Answer from the drawing. Dimensions are ordinates in mm from the lowest x, y and z of the part. Coordinates: 2 decimals unless noted, no trailing zeros. Write each loop counter-clockwise with the first axis right and the second up, starting at its lowest first coordinate (ties: lowest second). Pieces come first, ordered by that corner, then holes.
(1) The part is cut by section B-B, the plane z = 1.5. Determine the outline of the cut face in (x, y).
(2) The part is cut by section C-C, the plane y = 2.15. Determine the outline of the cut face in (x, z).
(3) Given pin 1 (8 mm diameter, centred on x = 18, z = 11.5, fed in from -Y); pin 2 (1.5 mm diameter, centred on x = 49, y = 1, fed in from -Z); pin 3 (0.9 mm diameter, centred on y = 1, z = 1, fed in from +X); pin 4 (1.5 mm diameter, centred on x = 16.5, y = 1.5, fed in from -Z), each flat-ended and moving along its own axis, determine where each tip first touches the part or whether it passes through.
(4) The part is cut by section D-D, the plane x = 25.4. Determine the outline of the cut face in (y, z), and give its area (3 significant figures).
(5) Straight lines are drawn through the part: line 1 along X through (y, z) = (1, 1.5); line 2 along Z through (x, y) = (49.3, 1.05); line 3 along X through (y, z) = (0.25, 4.25). For each, find the intervals that lie inside material, in ascending order.
(6) The part is cut by section A-A, the plane x = 49.3. Determine the outline of the cut face in (y, z), and give its area (3 significant figures).
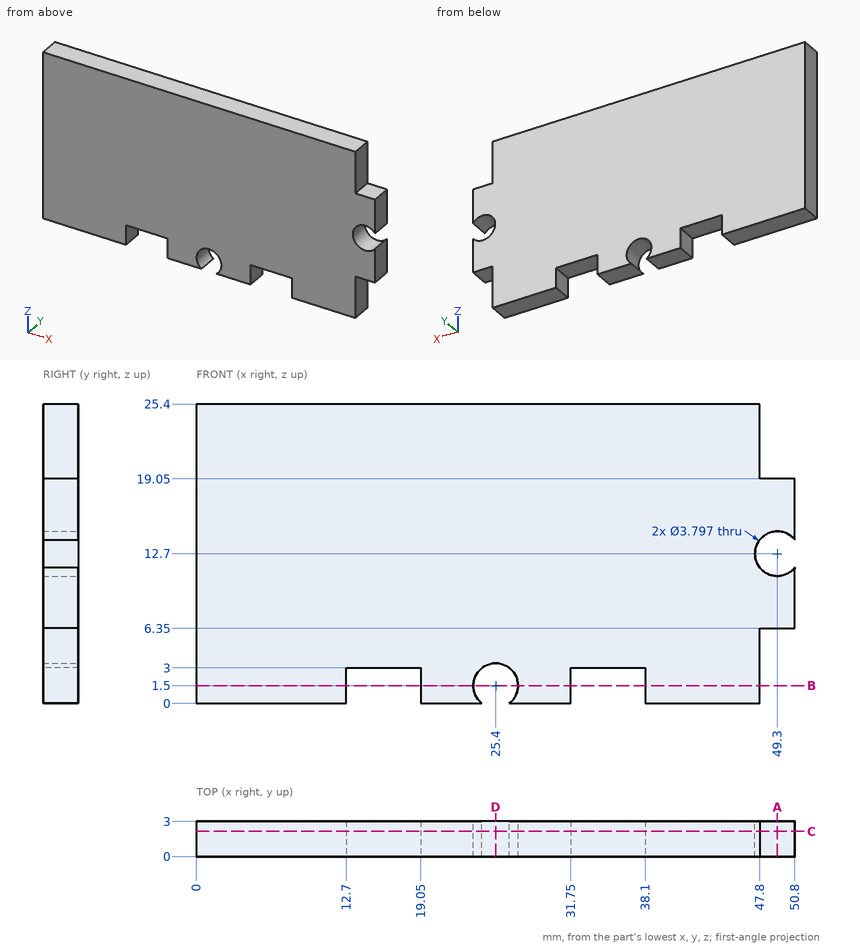
Computed:
1. outline: (0, 0) - (12.7, 0) - (12.7, 3) - (0, 3) - close; (19.05, 0) - (23.5, 0) - (23.5, 3) - (19.05, 3) - close; (27.3, 0) - (31.75, 0) - (31.75, 3) - (27.3, 3) - close; (38.1, 0) - (47.8, 0) - (47.8, 3) - (38.1, 3) - close
2. outline: (0, 0) - (12.7, 0) - (12.7, 3) - (19.05, 3) - (19.05, 0) - (24.24, 0) arc R1.9 cw (long way) to (26.56, 0) - (31.75, 0) - (31.75, 3) - (38.1, 3) - (38.1, 0) - (47.8, 0) - (47.8, 6.35) - (50.8, 6.35) - (50.8, 11.54) arc R1.9 cw (long way) to (50.8, 13.86) - (50.8, 19.05) - (47.8, 19.05) - (47.8, 25.4) - (0, 25.4) - close
3. pin 1: stops at y = 0
3. pin 2: stops at z = 6.35
3. pin 3: stops at x = 47.8
3. pin 4: stops at z = 3
4. outline: (0, 3.4) - (3, 3.4) - (3, 25.4) - (0, 25.4) - close
4. area: 66.0 mm2
5. line 1: x = 0 to 12.7, 19.05 to 23.5, 27.3 to 31.75, 38.1 to 47.8
5. line 2: z = 6.35 to 10.8, 14.6 to 19.05
5. line 3: x = 0 to 47.8
6. outline: (0, 6.35) - (3, 6.35) - (3, 10.8) - (0, 10.8) - close; (0, 14.6) - (3, 14.6) - (3, 19.05) - (0, 19.05) - close
6. area: 26.7 mm2
